```python
from build123d import *

# Parameters (mm, degrees)
SALIENTE_EXTRUIR1_DEPTH = 38.1
CORTAR_EXTRUIR18_DEPTH  = 38.1
CROQUIS4_OUTSIDE_W      = 580.479
CROQUIS4_OUTSIDE_H      = 149.876
CROQUIS4_OUTSIDE_R      = 19.177
CORTAR_EXTRUIR21_DEPTH  = 50.8


with BuildPart() as part:
    # Croquis1 → Saliente-Extruir1 (new body)
    with BuildSketch(Plane(origin=(0, 0, 0), x_dir=(1, 0, 0), z_dir=(0, 1, 0))):
        with BuildLine():
            Line((-61.958802083, 0), (369.841197917, 0))
            ThreePointArc((369.841197917, 0), (392.72185746, 26.5666935), (367.322364583, 50.7365))
            Line((367.322364583, 50.7365), (-64.477635417, 50.7365))
            ThreePointArc((-64.477635417, 50.7365), (-88.58646875, 24.108833333), (-61.958802083, 0))
        make_face()
    extrude(amount=SALIENTE_EXTRUIR1_DEPTH)

    # Croquis3 → Cortar-Extruir18 (cut)
    with BuildSketch(Plane(origin=(0, 38.1, 0), x_dir=(1, 0, 0), z_dir=(0, 1, 0))):
        with BuildLine():
            add(Edge.make_bspline(
                [(68.053382641, 25.36825), (85.128897701, 37.242607365), (117.715779547, 53.529246636), (147.710358419, 35.418129568), (159.94527156, 27.422727745)],
                knots=[0.293668056, 0.293668056, 0.293668056, 0.293668056, 0.509999468, 0.663692502, 0.663692502, 0.663692502, 0.663692502], degree=3))
            add(Edge.make_bspline(
                [(68.053382641, 25.36825), (85.297187869, 13.221681932), (118.362782549, -4.355831371), (146.208725565, 18.171330049), (158.923925731, 26.746070777), (159.94527156, 27.422727745)],
                knots=[0.293535528, 0.293535528, 0.293535528, 0.293535528, 0.509769313, 0.658147643, 0.671041491, 0.671041491, 0.671041491, 0.671041491], degree=3))
        make_face()
    extrude(amount=-CORTAR_EXTRUIR18_DEPTH, mode=Mode.SUBTRACT)

    # Croquis4 outside → Cortar-Extruir21 (cut)
    # profile 1 of 3: a face of its own
    with BuildSketch(Plane(origin=(0, 38.1, 0), x_dir=(1, 0, 0), z_dir=(0, 1, 0))):
        with Locations((152.0675, 25.353)):
            Rectangle(CROQUIS4_OUTSIDE_W, CROQUIS4_OUTSIDE_H)
        with BuildLine():
            Line((-64.477635417, 50.7365), (367.322364583, 50.7365))
            ThreePointArc((367.322364583, 50.7365), (392.72185746, 26.5666935), (369.841197917, 0))
            Line((369.841197917, 0), (-61.958802083, 0))
            ThreePointArc((-61.958802083, 0), (-88.58646875, 24.108833333), (-64.477635417, 50.7365))
        make_face(mode=Mode.SUBTRACT)
    # profile 2 of 3: a face of its own
    with BuildSketch(Plane(origin=(0, 38.1, 0), x_dir=(1, 0, 0), z_dir=(0, 1, 0))):
        with Locations(Location((-63.21821875, 25.36825, 0), (0, 0, 270))):
            Circle(CROQUIS4_OUTSIDE_R)
    # profile 3 of 3: a face of its own
    with BuildSketch(Plane(origin=(0, 38.1, 0), x_dir=(1, 0, 0), z_dir=(0, 1, 0))):
        with Locations(Location((367.322364583, 25.305725768, 0), (0, 0, 270))):
            Circle(CROQUIS4_OUTSIDE_R)
    extrude(amount=-CORTAR_EXTRUIR21_DEPTH, mode=Mode.SUBTRACT)


solid = part.part
```
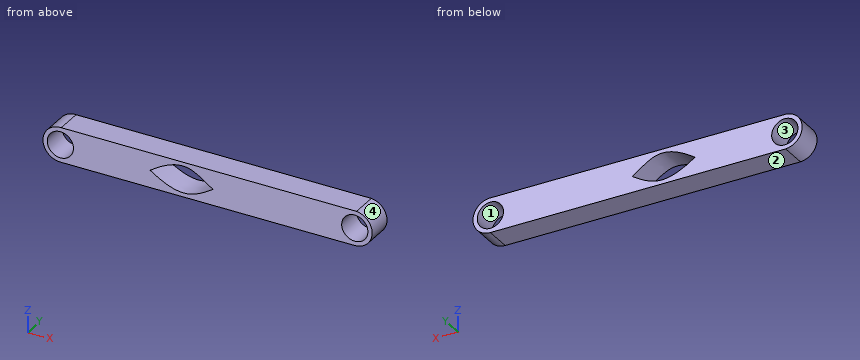
CAD build for the part. Positions are in the model's coordinates, mm. Face numbers are marked on the shaded views. Round coordinates to 2 decimals unless told otherwise and drop trailing zeros. Loops run counter-clockwise (first coordinate to the right, second up) from the corner with the lowest first, then second, coordinate; pieces in that order, holes last. Notation, with made-up numbers: M 24,17.25 L 37,17.25 A23 cw 37,27.25 Z; hole C -4.75,83 d1. An arc over 180 degrees is marked long. Return JSON: item names as keys, results as strings. Group by question number.
(1) Mould opens along X. For the marked faces 1, 2, 3 and 4 say: +X half, -X half, draft (parallel to the pull), parting line (faces both ways), or undercut.
(2) Drop flat-ended pins along their axis: P1, Ø4, axis at x = 179.5, y = 28, coming from the +Z side; P2, Ø5, axis at x = 114, z = -10.5, coming from the -Y side; P3, Ø6, axis at y = 14.5, z = -17, coming from the +X side; P4, Ø2, axis at y = 32.5, z = -30.5, coming from the -X side. Give the stop position or say it passes through.
(3) Wall check: probe 1 along X at (y, z) = (21.5, -38); probe 2 along Z at (x, y) = (-9.5, 11.5); probe 3 along X at (y, z) = (14.5, -29.5). Give the ranges that are in metal, low to high. Write a range as [from, to].
(4) Saw through at A-A, the plane x = -48. List the corners of the cut face in (y, z), and give its area (3 significant figures).
(5) Saw through at B-B, the plane z = -16.5. Give the number of separate pieces and of enclosed holes in the cut face, and give its area (3 significant figures).
Answer list:
{
 "1": {"face 1": "undercut", "face 2": "draft", "face 3": "undercut", "face 4": "+X half"},
 "2": {"P1": "z = 0", "P2": "through", "P3": "x = 392.19", "P4": "x = -88.28"},
 "3": {"probe 1": "[-85.25, -77.65], [-48.79, 89.55], [142.16, 352.95], [381.7, 389.36]", "probe 2": "[-50.74, 0]", "probe 3": "[-88.28, -81.94], [-44.49, 74.24], [156.74, 348.61], [386.04, 392.4]"},
 "4": {"outline": "M 0,-50.74 L 38.1,-50.74 L 38.1,-37.04 L 0,-37.04 Z; M 0,-13.7 L 38.1,-13.7 L 38.1,0 L 0,0 Z", "area": "1,040 mm2"},
 "5": {"separate pieces": "4", "enclosed holes": "0", "area": "13,300 mm2"}
}
